from build123d import *

# Parameters (mm, degrees)
ESQUISSE1_R        = 1.75
ESQUISSE1_R_2      = 1.35
BOSS_EXTRU_1_DEPTH = 6
CHANFREIN1_SIZE    = 1.25
CONG_1_R           = 10


with BuildPart() as part:
    # Esquisse1 → Boss.-Extru.1 (new body)
    with BuildSketch(Plane.XY):
        with BuildLine():
            Line((113.453134084, 0), (121, 0))
            ThreePointArc((121, 0), (126, 5), (121, 10))
            Line((121, 10), (108, 10))
            ThreePointArc((108, 10), (81.5, -5.93763889), (55, 10))
            Line((55, 10), (0, 10))
            ThreePointArc((0, 10), (-5, 5), (0, 0))
            Line((0, 0), (49.546865916, 0))
            ThreePointArc((49.546865916, 0), (81.5, -15.93763889), (113.453134084, 0))
        make_face()
        with Locations((0, 5)):
            Circle(ESQUISSE1_R, mode=Mode.SUBTRACT)
        with Locations((121, 5)):
            Circle(ESQUISSE1_R_2, mode=Mode.SUBTRACT)
    extrude(amount=BOSS_EXTRU_1_DEPTH)

    # Chanfrein1
    chanfrein1_edges = [part.edges().sort_by_distance(p)[0] for p in [
        (-1.75, 5, 0),
    ]]
    chamfer(chanfrein1_edges, length=CHANFREIN1_SIZE)

    # Congé1
    cong_1_edges = [part.edges().sort_by_distance(p)[0] for p in [
        (55, 10, 3),
        (108, 10, 3),
        (113.453134084, 0, 3),
        (49.546865916, 0, 3),
    ]]
    fillet(cong_1_edges, radius=CONG_1_R)


solid = part.part
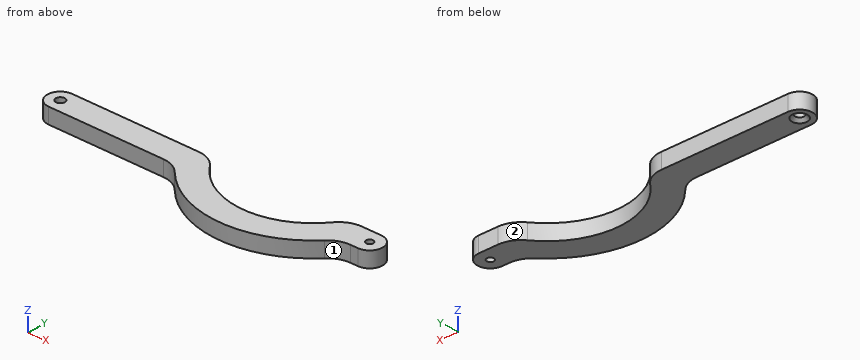
Design review of the part built by this model. Coordinates are the model's own, in mm. Face numbers are marked on the shaded views. A direction names the side the tool comes from. Coordinates: 2 decimals unless noted, no trailing zeros. Order: outer loops, then holes, each group sorted by start corner. A loop starts at its lowest first (then second) coordinate and runs counter-clockwise, first axis right, second up. Notation, with made-up numbers: (34, 88) -> (87, 88) arc R21 ccw to (87, 92) -> close; hole circle Ø7 at (-29.5, 6). An arc over 180 degrees is marked (long way). One line per item, written item: value.
1) We need section B-B, the plane z = 3.05. Give the boundary of the cut face in (x, y).
Output values:
outline: (0, 0) -> (44.9, 0) arc R10 cw to (52.22, -3.19) arc R40 ccw to (110.78, -3.19) arc R10 cw to (118.1, 0) -> (121, 0) arc R5 ccw to (121, 10) -> (113.45, 10) arc R10 ccw to (105.46, 6.02) arc R30 cw to (57.54, 6.02) arc R10 ccw to (49.55, 10) -> (0, 10) arc R5 ccw to start; hole circle Ø3.5 at (0, 5); hole circle Ø2.7 at (121, 5)
2) Machinability: for the marked faces 1 and 2, which of the approach directions +Z, -Z, +X, -X, +Y, -Y give a long, thin tool a straight path to every point of the face, cutting with its end or side? Answer none if there is none.
Output values:
face 1: +Z, -Z, +X, -Y
face 2: +Z, -Z, +Y
3) We need section C-C, the plane x = 4.5. Give the boundary of the cut face in (y, z), then the cut area to 3 significant figures.
Output values:
outline: (0, 0) -> (10, 0) -> (10, 6) -> (0, 6) -> close
area: 60.0 mm2
4) We need section A-A, the plane y = -4.5. Give the boundary of the cut face in (x, z), then the cut area to 3 significant figures.
Output values:
outline: (53.5, 0) -> (72.32, 0) -> (72.32, 6) -> (53.5, 6) -> close; (90.68, 0) -> (109.5, 0) -> (109.5, 6) -> (90.68, 6) -> close
area: 226 mm2
5) We need section D-D, the plane x = 69.5. Give the boundary of the cut face in (y, z), then the cut area to 3 significant figures.
Output values:
outline: (-14.1, 0) -> (-3.43, 0) -> (-3.43, 6) -> (-14.1, 6) -> close
area: 64.0 mm2
6) To check wall thickness, follow probe 1 along Y at (x, z) = (0, 2.9); probe 2 along Y at (x, z) = (121, 1.8); probe 3 along Y at (x, z) = (44.5, 5.2). State the ranges of each line that lie inside material, in increasing order. Write a range as [from, to].
Output values:
probe 1: y = [0, 3.25], [6.75, 10]
probe 2: y = [0, 3.65], [6.35, 10]
probe 3: y = [0, 10]
7) Clearance check with flat-ended pins moving along their axes: P1, Ø3, axis at x = 26.5, z = 2, coming from the -Y side; P2, Ø3.5, axis at x = 121, y = 5, coming from the +Z side. State where each tip first meets the part, or that it passes through.
Output values:
P1: stops at y = 0
P2: stops at z = 6
